from build123d import *

# Parameters (mm, degrees)
SKETCH_1_W      = 50
SKETCH_1_H      = 10
SKETCH_1_R      = 2
EXTRUDE_1_DEPTH = 5
FILLET_1_R      = 5


with BuildPart() as part:
    # 草图1 → 凸台-拉伸1 (new body)
    with BuildSketch(Plane.XY):
        Rectangle(SKETCH_1_W, SKETCH_1_H)
        with Locations((-15, 0)):
            Circle(SKETCH_1_R, mode=Mode.SUBTRACT)
        with Locations(Location((15, 0, 0), (0, 0, 180))):
            Circle(SKETCH_1_R, mode=Mode.SUBTRACT)
        Circle(SKETCH_1_R, mode=Mode.SUBTRACT)
    extrude(amount=EXTRUDE_1_DEPTH)

    # 圆角1
    fillet_1_edges = [part.edges().sort_by_distance(p)[0] for p in [
        (25, -5, 2.5),
        (25, 5, 2.5),
        (-25, -5, 2.5),
        (-25, 5, 2.5),
    ]]
    fillet(fillet_1_edges, radius=FILLET_1_R - 0.0001)  # a hair under: the kernel refuses the full size


solid = part.part
Build history of the part. All positions in model axes, mm. Coordinates: 2 decimals unless noted, no trailing zeros. Order: outer loops, then holes, each group sorted by start corner. A loop starts at its lowest first (then second) coordinate and runs counter-clockwise, first axis right, second up. Notation, with made-up numbers: (-23.75, 1.5) - (3.25, 1.5) arc R28 ccw to (3.25, 37.5) - close; hole circle Ø7 at (-31, -34). An arc over 180 degrees is marked (long way). Write each question's results on one line, items separated by ' | '. Start each with the question number.
Item 1: Wall check: probe 1 along Y at (x, z) = (-15, 1.65); probe 2 along X at (y, z) = (-1.25, 2.6); probe 3 along X at (y, z) = (0.5, 1.4). Give the ranges that are in metal, low to high. Write a range as [from, to].
Item 2: Mould opens along X. For faces 1 (the face through (16.6, 1.2, 2.5)), 2 (the face through (-24, -3, 3)), 3 (the face through (0, -2, 2)), 4 (the face through (23, -4, 3)) say: released by +X, released by -X, zero draft, split by the parting line, or undercut.
Item 3: Band-saw the part on C-C on y = 0.75. Write the cut outline in (x, z), and give its area (3 significant figures).
Item 4: Flat gauge pins, fed straight in: pin 1 (3 mm diameter, centred on y = -0.5, z = 3, fed in from +X); pin 2 (1 mm diameter, centred on y = -3, z = 1, fed in from -X). Where does each tip first touch, or does it go through?
Item 5: Band-saw the part on B-B on x = 15. Write the cut outline in (y, z), and give its area (3 significant figures).
Item 6: Band-saw the part on D-D on y = 4. Write the cut outline in (x, z).
Item 7: Band-saw the part on A-A on z = 1.2. State how many separate pieces and enclosed holes the cut face has, and give its area (3 significant figures).
Numbers:
1) probe 1: [-5, -2], [2, 5] | probe 2: [-24.84, -16.56], [-13.44, -1.56], [1.56, 13.44], [16.56, 24.84] | probe 3: [-24.97, -16.94], [-13.06, -1.94], [1.94, 13.06], [16.94, 24.97]
2) face 1: undercut | face 2: released by -X | face 3: undercut | face 4: released by +X
3) outline: (-24.94, 0) - (-16.85, 0) - (-16.85, 5) - (-24.94, 5) - close; (-13.15, 0) - (-1.85, 0) - (-1.85, 5) - (-13.15, 5) - close; (1.85, 0) - (13.15, 0) - (13.15, 5) - (1.85, 5) - close; (16.85, 0) - (24.94, 0) - (24.94, 5) - (16.85, 5) - close | area: 194 mm^2
4) pin 1: x = 25 | pin 2: x = -24.33
5) outline: (-5, 0) - (-2, 0) - (-2, 5) - (-5, 5) - close; (2, 0) - (5, 0) - (5, 5) - (2, 5) - close | area: 30.0 mm^2
6) outline: (-23, 0) - (23, 0) - (23, 5) - (-23, 5) - close
7) separate pieces: 1 | enclosed holes: 3 | area: 441 mm^2
